Source: three-view drawing plus pictorial views. Frame: mm from the lowest corner of the part. Give positions to 0.01 mm unless a question says otherwise; leave off trailing zeros. Order: outer loops, then holes, each group sorted by start corner. A loop starts at its lowest first (then second) coordinate and runs counter-clockwise, first axis right, second up. Notation, with made-up numbers: (28, 65) -> (72, 65) arc R8 cw to (72, 80) -> close; hole circle Ø2 at (54.5, 58). An arc over 180 degrees is marked (long way). Answer in a Markdown table with one row per item.
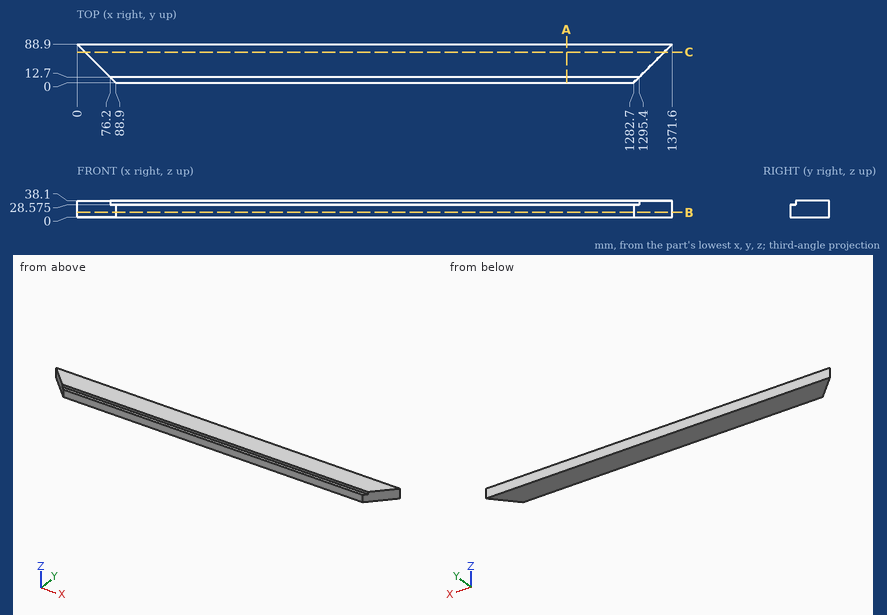
(1) First-contact query: pin 1 Ø1 at (y, z) = (55, 7) entering from +X; pin 2 Ø6.5 at (x, y) = (699, 4) entering from +Z (3 decimals); pin 3 Ø10 at (y, z) = (37.5, 12.5) entering from -X. Flat tips, straight axial feed; report the tip coordinate or a pass-through.
A:
| item | result |
|---|---|
| pin 1 | stops at x = 1338.2 |
| pin 2 | stops at z = 28.575 |
| pin 3 | stops at x = 46.4 |
(2) Section query A-A (x = 1128). Return the cut outline in (y, z) (3 decimals).
A:
| item | result |
|---|---|
| outline | (0, 0) -> (88.9, 0) -> (88.9, 38.1) -> (12.7, 38.1) -> (12.7, 28.575) -> (0, 28.575) -> close |
(3) Ray query, probe 1 along Z at (x, y) = (1187, 6.5) (3 decimals); probe 2 along X at (y, z) = (25, 32.5); probe 3 along Y at (x, z) = (79.5, 26.5). Return the intervals inside material, ascending.
A:
| item | result |
|---|---|
| probe 1 | z = 0 to 28.575 |
| probe 2 | x = 63.9 to 1307.7 |
| probe 3 | y = 9.4 to 88.9 |
(4) Section query B-B (z = 11). Return the cut outline in (x, y).
A:
| item | result |
|---|---|
| outline | (0, 88.9) -> (88.9, 0) -> (1282.7, 0) -> (1371.6, 88.9) -> close |
(5) Section query C-C (y = 70). Return the cut outline in (x, z).
A:
| item | result |
|---|---|
| outline | (18.9, 0) -> (1352.7, 0) -> (1352.7, 38.1) -> (18.9, 38.1) -> close |
